Geometry check sheet. Reference: the model listing, model coordinates, mm. A direction names the side the tool comes from. Give positions to 0.01 mm unless a question says otherwise; leave off trailing zeros. Order: outer loops, then holes, each group sorted by start corner. A loop starts at its lowest first (then second) coordinate and runs counter-clockwise, first axis right, second up. Notation, with made-up numbers: M 58.5,14 L 92.5,14 A18 ccw 92.5,20 Z; hole C -9,84 d5. An arc over 180 degrees is marked long. Answer as a JSON object with one key per item and string values. Group by question number.
from build123d import *

# Parameters (mm, degrees)
F0_R         = 25
F1_DEPTH     = 10
F2_R         = 7.5
F3_DEPTH     = 10.001
F4_R         = 17.5
F5_DEPTH     = 10
F6_R         = 4
F7_DEPTH     = 20
F8_R         = 2.25
F9_DEPTH     = 24.4801666667
F10_W        = 7.2
F10_H        = 3.5
F11_DEPTH    = 9.2
F13_R        = 3.75
F14_DEPTH    = 13.5
F15_C1_SIZE  = 2
F15_C2_SIZE  = 2
F15_C3_SIZE  = 2
F15_C4_SIZE  = 2
F15_C5_SIZE  = 2
F15_C6_SIZE  = 2
F15_C7_SIZE  = 2
F15_C8_SIZE  = 2
F15_C9_SIZE  = 2
F15_C10_SIZE = 2
F15_C11_SIZE = 2
F15_C12_SIZE = 2
F15_C13_SIZE = 2
F15_C14_SIZE = 2
F15_C15_SIZE = 2
F15_C16_SIZE = 2
F15_C17_SIZE = 2
F15_C18_SIZE = 2
F15_C19_SIZE = 2
F15_C20_SIZE = 2
F15_C21_SIZE = 2
F15_C22_SIZE = 2
F15_C23_SIZE = 2


with BuildPart() as f1:
    # F0 (on Top) → F1 (new body)
    with BuildSketch(Plane.XY):
        Circle(F0_R)
    extrude(amount=F1_DEPTH)

    # F2 (on face) → F3 (cut, through all)
    with BuildSketch(Plane.XY.offset(10)):
        with Locations((0, 30)):
            Circle(F2_R)
        with Locations((-15, 25.9807621135)):
            Circle(F2_R)
        with Locations((-25.9807621135, 15)):
            Circle(F2_R)
        with Locations((-30, 0)):
            Circle(F2_R)
        with Locations((-25.9807621135, -15)):
            Circle(F2_R)
        with Locations((-15, -25.9807621135)):
            Circle(F2_R)
        with Locations((0, -30)):
            Circle(F2_R)
        with Locations((15, -25.9807621135)):
            Circle(F2_R)
        with Locations((25.9807621135, -15)):
            Circle(F2_R)
        with Locations((30, 0)):
            Circle(F2_R)
        with Locations((25.9807621135, 15)):
            Circle(F2_R)
        with Locations((15, 25.9807621135)):
            Circle(F2_R)
    extrude(amount=-F3_DEPTH, mode=Mode.SUBTRACT)

    # F4 (on face) → F5 (join)
    with BuildSketch(Plane.XY.offset(10)):
        Circle(F4_R)
    extrude(amount=F5_DEPTH)

    # F6 (on face) → F7 (cut, through all)
    with BuildSketch(Plane.XY.offset(20)):
        Circle(F6_R)
    extrude(amount=-F7_DEPTH, mode=Mode.SUBTRACT)

    # F8 (on Front) → F9 (cut, through all)
    with BuildSketch(Plane.XZ):
        with Locations((0, 15)):
            Circle(F8_R)
    extrude(amount=-F9_DEPTH, mode=Mode.SUBTRACT)

    # F10 (on face) → F11 (cut)
    with BuildSketch(Plane.XY.offset(20)):
        with Locations((0, 7.75)):
            Rectangle(F10_W, F10_H)
    extrude(amount=-F11_DEPTH, mode=Mode.SUBTRACT)

    # F13 (on offset) → F14 (cut, through all)
    with BuildSketch(Plane.XZ.offset(-25)):
        with Locations((0, 15)):
            Circle(F13_R)
    extrude(amount=F14_DEPTH, mode=Mode.SUBTRACT)

    # F15: chamfer of 2 on 23 edges, made by hand

    # F15_c1
    f15_c1_edges = [f1.edges().sort_by_distance(p)[0] for p in [
        (24.1481456572, 6.4704761276, 0),
    ]]
    chamfer(f15_c1_edges, length=F15_C1_SIZE)

    # F15_c2
    f15_c2_edges = [f1.edges().sort_by_distance(p)[0] for p in [
        (22.6680317958, -1.5786837087, 0),
    ]]
    chamfer(f15_c2_edges, length=F15_C2_SIZE)

    # F15_c3
    f15_c3_edges = [f1.edges().sort_by_distance(p)[0] for p in [
        (23.8267406055, -7.5687800944, 0),
    ]]
    chamfer(f15_c3_edges, length=F15_C3_SIZE)

    # F15_c4
    f15_c4_edges = [f1.edges().sort_by_distance(p)[0] for p in [
        (18.8417495346, 12.7011960942, 0),
    ]]
    chamfer(f15_c4_edges, length=F15_C4_SIZE)

    # F15_c5
    f15_c5_edges = [f1.edges().sort_by_distance(p)[0] for p in [
        (18.8417495346, -12.7011960942, 0),
    ]]
    chamfer(f15_c5_edges, length=F15_C5_SIZE)

    # F15_c6
    f15_c6_edges = [f1.edges().sort_by_distance(p)[0] for p in [
        (16.8501726066, 18.4681261401, 0),
    ]]
    chamfer(f15_c6_edges, length=F15_C6_SIZE)

    # F15_c7
    f15_c7_edges = [f1.edges().sort_by_distance(p)[0] for p in [
        (16.8501726066, -18.4681261401, 0),
    ]]
    chamfer(f15_c7_edges, length=F15_C7_SIZE)

    # F15_c8
    f15_c8_edges = [f1.edges().sort_by_distance(p)[0] for p in [
        (9.9668357016, 20.4204332433, 0),
    ]]
    chamfer(f15_c8_edges, length=F15_C8_SIZE)

    # F15_c9
    f15_c9_edges = [f1.edges().sort_by_distance(p)[0] for p in [
        (9.9668357016, -20.4204332433, 0),
    ]]
    chamfer(f15_c9_edges, length=F15_C9_SIZE)

    # F15_c10
    f15_c10_edges = [f1.edges().sort_by_distance(p)[0] for p in [
        (5.3586144654, 24.418952701, 0),
    ]]
    chamfer(f15_c10_edges, length=F15_C10_SIZE)

    # F15_c11
    f15_c11_edges = [f1.edges().sort_by_distance(p)[0] for p in [
        (5.3586144654, -24.418952701, 0),
    ]]
    chamfer(f15_c11_edges, length=F15_C11_SIZE)

    # F15_c12
    f15_c12_edges = [f1.edges().sort_by_distance(p)[0] for p in [
        (-1.5786837087, 22.6680317958, 0),
    ]]
    chamfer(f15_c12_edges, length=F15_C12_SIZE)

    # F15_c13
    f15_c13_edges = [f1.edges().sort_by_distance(p)[0] for p in [
        (-1.5786837087, -22.6680317958, 0),
    ]]
    chamfer(f15_c13_edges, length=F15_C13_SIZE)

    # F15_c14
    f15_c14_edges = [f1.edges().sort_by_distance(p)[0] for p in [
        (-7.5687800944, 23.8267406055, 0),
    ]]
    chamfer(f15_c14_edges, length=F15_C14_SIZE)

    # F15_c15
    f15_c15_edges = [f1.edges().sort_by_distance(p)[0] for p in [
        (-7.5687800944, -23.8267406055, 0),
    ]]
    chamfer(f15_c15_edges, length=F15_C15_SIZE)

    # F15_c16
    f15_c16_edges = [f1.edges().sort_by_distance(p)[0] for p in [
        (-12.7011960942, 18.8417495346, 0),
    ]]
    chamfer(f15_c16_edges, length=F15_C16_SIZE)

    # F15_c17
    f15_c17_edges = [f1.edges().sort_by_distance(p)[0] for p in [
        (-12.7011960942, -18.8417495346, 0),
    ]]
    chamfer(f15_c17_edges, length=F15_C17_SIZE)

    # F15_c18
    f15_c18_edges = [f1.edges().sort_by_distance(p)[0] for p in [
        (-18.4681261401, 16.8501726066, 0),
    ]]
    chamfer(f15_c18_edges, length=F15_C18_SIZE)

    # F15_c19
    f15_c19_edges = [f1.edges().sort_by_distance(p)[0] for p in [
        (-18.4681261401, -16.8501726066, 0),
    ]]
    chamfer(f15_c19_edges, length=F15_C19_SIZE)

    # F15_c20
    f15_c20_edges = [f1.edges().sort_by_distance(p)[0] for p in [
        (-20.4204332433, 9.9668357016, 0),
    ]]
    chamfer(f15_c20_edges, length=F15_C20_SIZE)

    # F15_c21
    f15_c21_edges = [f1.edges().sort_by_distance(p)[0] for p in [
        (-20.4204332433, -9.9668357016, 0),
    ]]
    chamfer(f15_c21_edges, length=F15_C21_SIZE)

    # F15_c22
    f15_c22_edges = [f1.edges().sort_by_distance(p)[0] for p in [
        (-24.418952701, -5.3586144654, 0),
    ]]
    chamfer(f15_c22_edges, length=F15_C22_SIZE)

    # F15_c23
    f15_c23_edges = [f1.edges().sort_by_distance(p)[0] for p in [
        (-22.6680317958, 1.5786837087, 0),
    ]]
    chamfer(f15_c23_edges, length=F15_C23_SIZE)


solid = f1.part
1. Thickness scan on line 1 along Z through (x, y) = (0, 16.25); line 2 along Y through (x, z) = (0, 9.5); line 3 along X through (y, z) = (-2.5, 18). Record the ranges inside material, lowest first. Write a range as [from, to].
2. Cross-section at B-B (x = 0). State how many separate pieces and enclosed holes the cut face has, and give its area (3 significant figures).
3. Depth check by flat-ended pin: pin 1 (8.5 mm diameter, centred on x = 0, z = 15, fed in from +Y); pin 2 (4 mm diameter, centred on y = 7.5, z = 17, fed in from -X); pin 3 (1 mm diameter, centred on x = 4, y = 19.5, fed in from -Z); pin 4 (5 mm diameter, centred on x = 0, z = 15, fed in from -Y). Enter the tip coordinate at first touch or a pass-through.
4. Cross-section at A-A (y = 0). Record the cut outline in (x, z), and give its area (3 significant figures).
5. Release check for a two-part mould opening along Y. For faces 4 (the cylindrical face through (-0.867, -3.905, 10.14)), 5 (the cylindrical face through (19.447, 11.318, 6.056)), 6 (the conical face through (23.41, -6.29, 1.24)), 7 (the cylindrical face through (-11.318, 19.447, 6.056)) record: released by +Y, released by -Y, zero draft, split by the parting line, or undercut.
6. Access from +Z, -Z, +X, -X, +Y, -Y to the whole of each face (thin tool, end or side, straight path). Record for faces 1 (the cylindrical face through (-24.153, -6.451, 5.944)), 2 (the flat face through (-3.6, 8, 15)), 3 (the flat face through (2, 11.5, 13)).
7. Cross-section at C-C (z = 5.25). Record the cut outline in (x, y).
8. Cross-section at D-D (z = 12). Record the cut outline in (x, y), and give its area (3 significant figures).
Report:
{
 "1": {"line 1": "z = [0, 11.25], [18.75, 20]", "line 2": "y = [-22.5, -4], [4, 22.5]", "line 3": "x = [-17.32, -3.12], [3.12, 17.32]"},
 "2": {"separate pieces": "4", "enclosed holes": "0", "area": "541 mm2"},
 "3": {"pin 1": "stops at y = 17.5", "pin 2": "stops at x = -16.61", "pin 3": "stops at z = 0", "pin 4": "stops at y = -17.5"},
 "4": {"outline": "M -22.5,2 L -20.5,0 L -4,0 L -4,20 L -17.5,20 L -17.5,10 L -22.5,10 Z; M 4,0 L 20.5,0 L 22.5,2 L 22.5,10 L 17.5,10 L 17.5,20 L 4,20 Z", "area": "636 mm2"},
 "5": {"face 4": "undercut", "face 5": "undercut", "face 6": "released by -Y", "face 7": "released by +Y"},
 "6": {"face 1": "+Z, -Z, -X, -Y", "face 2": "+Z", "face 3": "+Y"},
 "7": {"outline": "M -24.48,-5.08 A25 ccw -23.74,-7.84 A7.5 cw -18.66,-16.64 A25 ccw -16.64,-18.66 A7.5 cw -7.84,-23.74 A25 ccw -5.08,-24.48 A7.5 cw 5.08,-24.48 A25 ccw 7.84,-23.74 A7.5 cw 16.64,-18.66 A25 ccw 18.66,-16.64 A7.5 cw 23.74,-7.84 A25 ccw 24.48,-5.08 A7.5 cw 24.48,5.08 A25 ccw 23.74,7.84 A7.5 cw 18.66,16.64 A25 ccw 16.64,18.66 A7.5 cw 7.84,23.74 A25 ccw 5.08,24.48 A7.5 cw -5.08,24.48 A25 ccw -7.84,23.74 A7.5 cw -16.64,18.66 A25 ccw -18.66,16.64 A7.5 cw -23.74,7.84 A25 ccw -24.48,5.08 A7.5 cw Z; hole C 0,0 d8"},
 "8": {"outline": "M -2.25,11.5 L -2.25,17.35 A17.5 ccw long 2.25,17.35 L 2.25,11.5 Z; hole C 0,0 d8; hole M -3.6,6 L 3.6,6 L 3.6,9.5 L -3.6,9.5 Z", "area": "860 mm2"}
}
